Study the drawing (mm; zero at the part's minimum x, y, z) and answer. Give positions to 0.01 mm unless a question says otherwise; leave off trailing zeros. Loops run counter-clockwise (first coordinate to the right, second up) from the corner with the lowest first, then second, coordinate; pieces in that order, holes last. Notation, with made-up numbers: (18, 20.25) - (56, 20.25) arc R17 cw to (56, 46.25) - close; hole circle Ø4 at (-23, -4.75). An arc over 180 degrees is marked (long way). One line per item, written item: value. Start each with the question number.
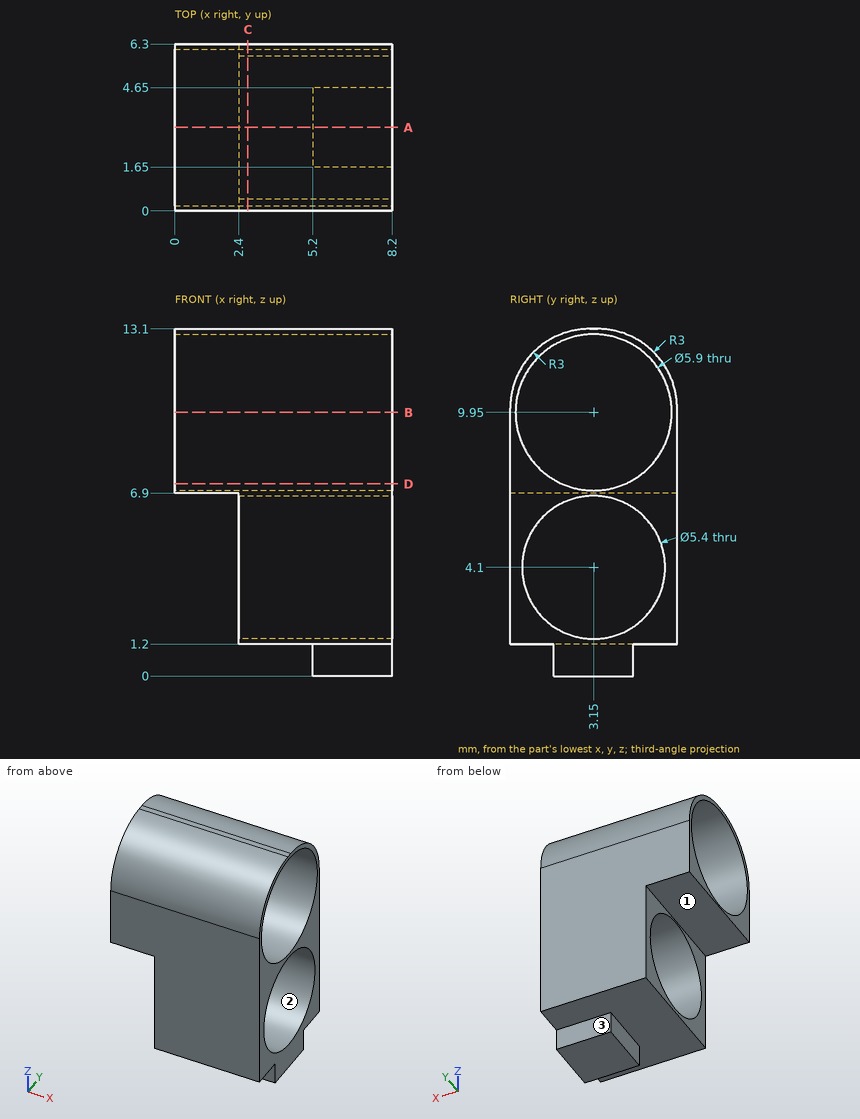
1. Flat-ended cylindrical pins translate along their axes: pin 1 (0.7 mm diameter, centred on x = 1, y = 4.5, fed in from -Z); pin 2 (0.6 mm diameter, centred on y = 3.5, z = 1, fed in from -X); pin 3 (3 mm diameter, centred on x = 2, y = 3.5, fed in from -Z); pin 4 (3 mm diameter, centred on y = 1.5, z = 3, fed in from +X). Find the tip coordinate at first contact, or state that the pin passes through.
2. Find the intervals of material crossed by L1, parallel to Y at x = 4.1, z = 4.1; L2, parallel to Y at x = 4, z = 9.95; L3, parallel to Z at x = 6.5, y = 2, in increasing order. Write a range as [from, to].
3. A cutting plane is placed at B-B (z = 9.95). Determine the outline of the cut face in (x, y), plus the area to 3 significant figures.
4. A cutting plane is placed at C-C (x = 2.75). Determine the outline of the cut face in (y, z).
5. Determine the mould class of the marked faces 1, 2 and 3 for opening direction Y: released by +Y, released by -Y, zero draft, split by the parting line, or undercut.
6. A cutting plane is placed at A-A (y = 3.15). Determine the outline of the cut face in (x, z).
7. A cutting plane is placed at D-D (z = 7.25). Determine the outline of the cut face in (x, y).
Results below:
1. pin 1: stops at z = 6.9
1. pin 2: stops at x = 2.4
1. pin 3: stops at z = 1.2
1. pin 4: stops at x = 8.2
2. L1: y = [0, 0.45], [5.85, 6.3]
2. L2: y = [0, 0.2], [6.1, 6.3]
2. L3: z = [0, 1.66], [6.54, 7.23], [12.67, 12.93]
3. outline: (0, 0) - (8.2, 0) - (8.2, 0.2) - (0, 0.2) - close; (0, 6.1) - (8.2, 6.1) - (8.2, 6.3) - (0, 6.3) - close
3. area: 3.28 mm^2
4. outline: (0, 1.2) - (6.3, 1.2) - (6.3, 10.1) arc R3 ccw to (3.3, 13.1) - (3, 13.1) arc R3 ccw to (0, 10.1) - close; hole circle Ø5.9 at (3.15, 9.95); hole circle Ø5.4 at (3.15, 4.1)
5. face 1: zero draft
5. face 2: undercut
5. face 3: released by +Y
6. outline: (0, 6.9) - (2.4, 6.9) - (2.4, 6.8) - (8.2, 6.8) - (8.2, 7) - (0, 7) - close; (0, 12.9) - (8.2, 12.9) - (8.2, 13.1) - (0, 13.1) - close; (2.4, 1.2) - (5.2, 1.2) - (5.2, 0) - (8.2, 0) - (8.2, 1.4) - (2.4, 1.4) - close
7. outline: (0, 0) - (8.2, 0) - (8.2, 1.96) - (0, 1.96) - close; (0, 4.34) - (8.2, 4.34) - (8.2, 6.3) - (0, 6.3) - close
